Read the model definition and answer for the solid it produces. Units are mm, in the model's axes. A direction names the side the tool comes from. Give positions to 0.01 mm unless a question says otherwise; leave off trailing zeros. Write each loop counter-clockwise with the first axis right and the second up, starting at its lowest first coordinate (ties: lowest second). Pieces come first, ordered by that corner, then holes. Notation, with made-up numbers: M 56,76 L 104,76 A22 cw 104,102 Z; hole C 27.25,32.25 d8. An arc over 180 degrees is marked long. Put each result on its own line as item: value.
from build123d import *

# Parameters (mm, degrees)
SKETCH1_W                           = 22
SKETCH1_H                           = 28
BOSS_EXTRUDE1_DEPTH                 = 1.57
F_2_6_2_6_DIAMETER_HOLE1_AT_2_COUNT = 2
F_2_6_2_6_DIAMETER_HOLE1_AT_2_PITCH = 11
F_2_6_2_6_DIAMETER_HOLE1_AT_3_COUNT = 2
F_2_6_2_6_DIAMETER_HOLE1_AT_3_PITCH = 21.09502311
F_2_6_2_6_DIAMETER_HOLE1_AT_4_COUNT = 2
F_2_6_2_6_DIAMETER_HOLE1_AT_4_PITCH = 18
SKETCH5_W                           = 5
SKETCH5_H                           = 4.4
BOSS_EXTRUDE2_DEPTH                 = 1.2
SKETCH6_W                           = 21
SKETCH6_H                           = 3.08
BOSS_EXTRUDE3_DEPTH                 = 10


with BuildPart() as part:
    # Sketch1 → Boss-Extrude1 (new body)
    with BuildSketch(Plane(origin=(0, 0, 0), x_dir=(1, 0, 0), z_dir=(0, 1, 0))):
        with Locations((0, 6.5)):
            Rectangle(SKETCH1_W, SKETCH1_H)
    extrude(amount=BOSS_EXTRUDE1_DEPTH)

    # Sketch3 → Ø2.6 (2.6) Diameter Hole1 (revolve, cut)
    with BuildSketch(Plane(origin=(-9, 1.57, -5.5), x_dir=(0, 0, 1), z_dir=(1, 0, 0))):
        Polygon((0, 0), (0, 1.57), (1.325, 1.57), (1.3, 1.545), (1.3, 0), align=None)
    f_2_6_2_6_diameter_hole1 = revolve(axis=Axis((-9, 7.92, -5.5), (0, -1, 0)), mode=Mode.SUBTRACT)

    # Ø2.6 (2.6) Diameter Hole1 at 2: Ø2.6 (2.6) Diameter Hole1 ×2
    with Locations(*[(0, 0, i * F_2_6_2_6_DIAMETER_HOLE1_AT_2_PITCH) for i in range(1, F_2_6_2_6_DIAMETER_HOLE1_AT_2_COUNT)]):
        add(f_2_6_2_6_diameter_hole1, mode=Mode.SUBTRACT)

    # Ø2.6 (2.6) Diameter Hole1 at 3: Ø2.6 (2.6) Diameter Hole1 ×2
    with Locations(*[Vector(0.853281834, 0, 0.521450009) * (i * F_2_6_2_6_DIAMETER_HOLE1_AT_3_PITCH) for i in range(1, F_2_6_2_6_DIAMETER_HOLE1_AT_3_COUNT)]):
        add(f_2_6_2_6_diameter_hole1, mode=Mode.SUBTRACT)

    # Ø2.6 (2.6) Diameter Hole1 at 4: Ø2.6 (2.6) Diameter Hole1 ×2
    with Locations(*[(i * F_2_6_2_6_DIAMETER_HOLE1_AT_4_PITCH, 0, 0) for i in range(1, F_2_6_2_6_DIAMETER_HOLE1_AT_4_COUNT)]):
        add(f_2_6_2_6_diameter_hole1, mode=Mode.SUBTRACT)

    # Sketch5 → Boss-Extrude2 (add)
    with BuildSketch(Plane(origin=(0, 1.57, 0), x_dir=(1, 0, 0), z_dir=(0, 1, 0))):
        Rectangle(SKETCH5_W, SKETCH5_H)
    extrude(amount=BOSS_EXTRUDE2_DEPTH)

    # Sketch6 → Boss-Extrude3 (add)
    with BuildSketch(Plane(origin=(0, 1.57, 0), x_dir=(1, 0, 0), z_dir=(0, 1, 0))):
        with Locations((0, 18.46)):
            Rectangle(SKETCH6_W, SKETCH6_H)
    extrude(amount=BOSS_EXTRUDE3_DEPTH)


solid = part.part
(1) For a pull along X with two mould halves and no side action, classify faces 4 (the face through (-10.5, 6, -18)), 5 (the face through (9.5, 0.8, -4.3)), 6 (the face through (0, 11.57, -18)) as +X half, -X half, draft (parallel to the pull), parting line (faces both ways), or undercut.
Result:
face 4: -X half
face 5: undercut
face 6: draft
(2) Straight lines are drawn through the part: line 1 along Z through (x, y) = (-9, 0.95); line 2 along X through (y, z) = (0.8, -5.5); line 3 along Z through (x, y) = (-1, 7). For each, find the intervals that lie inside material, in ascending order. Write a range as from..to.
Result:
line 1: z = -20.5..-6.8, -4.2..4.2, 6.8..7.5
line 2: x = -11..-10.3, -7.7..7.7, 10.3..11
line 3: z = -20..-16.92
(3) Section D-D on x = -4 is taken. Determine the outline of the cut face in (y, z).
Result:
outline: M 0,-20.5 L 1.57,-20.5 L 1.57,-20 L 11.57,-20 L 11.57,-16.92 L 1.57,-16.92 L 1.57,7.5 L 0,7.5 Z
(4) Section A-A on x = -9 is taken. Determine the outline of the cut face in (y, z) (3 decimals).
Result:
outline: M 0,-20.5 L 1.57,-20.5 L 1.57,-20 L 11.57,-20 L 11.57,-16.92 L 1.57,-16.92 L 1.57,-6.8 L 0.025,-6.8 L 0,-6.825 Z; M 0,-4.175 L 0.025,-4.2 L 1.57,-4.2 L 1.57,4.2 L 0.025,4.2 L 0,4.175 Z; M 0,6.825 L 0.025,6.8 L 1.57,6.8 L 1.57,7.5 L 0,7.5 Z
(5) Section C-C on z = 5.5 is taken. Determine the outline of the cut face in (x, y) (3 decimals), and give its area (3 significant figures).
Result:
outline: M -11,0 L -10.325,0 L -10.3,0.025 L -10.3,1.57 L -11,1.57 Z; M -7.7,0.025 L -7.675,0 L 7.675,0 L 7.7,0.025 L 7.7,1.57 L -7.7,1.57 Z; M 10.3,0.025 L 10.325,0 L 11,0 L 11,1.57 L 10.3,1.57 Z
area: 26.4 mm²
(6) Given pin 1 Ø2.5 at (y, z) = (5.5, -19) entering from -X; pin 2 Ø4 at (x, z) = (-7.5, -7) entering from -Y; pin 3 Ø5 at (x, y) = (0.5, 7.5) entering from +Z; pin 4 Ø6 at (x, z) = (0.5, -5) entering from +Y, each flat-ended and moving along its own axis, determine where each tip first touches the part or whether it passes through.
Result:
pin 1: stops at x = -10.5
pin 2: stops at y = 0
pin 3: stops at z = -16.92
pin 4: stops at y = 2.77
(7) Which of the six approach directions +Z, -Z, +X, -X, +Y, -Y give full straight-line access (tool end or side, diameter ignored) to faces 1 (the face through (0, 6, -20)), 2 (the face through (0, 2, 2.2)), 3 (the face through (2.5, 2, 0))?
Result:
face 1: -Z, +X, -X, +Y
face 2: +Z, +X, -X, +Y
face 3: +Z, +X, +Y
(8) Section B-B on z = -18.25 is taken. Determine the outline of the cut face in (x, y).
Result:
outline: M -11,0 L 11,0 L 11,1.57 L 10.5,1.57 L 10.5,11.57 L -10.5,11.57 L -10.5,1.57 L -11,1.57 Z
